from build123d import *

# Parameters (mm, degrees)
SALIENTE_EXTRUIR1_DEPTH      = 5
SALIENTE_EXTRUIR1_DEPTH_BACK = 5
SALIENTE_EXTRUIR2_START      = 14
CROQUIS2_R                   = 5
SALIENTE_EXTRUIR2_DEPTH      = 10
CROQUIS4_W                   = 10
CROQUIS4_H                   = 2.771281292
SALIENTE_EXTRUIR3_DEPTH      = 18.9
CHAFL_N1_SIZE                = 1.2
CROQUIS5_R                   = 1.7
CORTAR_EXTRUIR1_DEPTH        = 33.252493444
CROQUIS2_4_R                 = 5
SALIENTE_EXTRUIR8_DEPTH      = 14
CHAFL_N2_SIZE                = 10
CHAFL_N2_SIZE_2              = 1.3
CORTAR_EXTRUIR2_DEPTH        = 31.412223535
CORTAR_EXTRUIR2_DEPTH_BACK   = 31.412223535


# Some blends are built 0.0001 mm under size
with BuildPart() as part:
    # Croquis1 → Saliente-Extruir1 (new, two sides: drawn at the far end of the back side and taken through both)
    with BuildSketch(Plane(origin=(0, 0, 0), x_dir=(0, 0, -1), z_dir=(1, 0, 0)).offset(-SALIENTE_EXTRUIR1_DEPTH_BACK)):
        Polygon((2.829016319, 4.9), (-2.829016319, 4.9), (-5.658032638, 0), (-2.829016319, -4.9), (2.829016319, -4.9), (5.658032638, 0), align=None)
        Polygon((2.886751346, 0), (1.443375673, 2.5), (-1.443375673, 2.5), (-2.886751346, 0), (-1.443375673, -2.5), (1.443375673, -2.5), align=None, mode=Mode.SUBTRACT)
    extrude(amount=SALIENTE_EXTRUIR1_DEPTH + SALIENTE_EXTRUIR1_DEPTH_BACK)



with BuildPart() as body_2:
    # Croquis2 → Saliente-Extruir2 (new body)
    with BuildSketch(Plane(origin=(0, 4.9, 0), x_dir=(1, 0, 0), z_dir=(0, 1, 0)).offset(SALIENTE_EXTRUIR2_START)):
        Polygon((0, 7.159143338), (-6.2, 3.579571669), (-6.2, -3.579571669), (0, -7.159143338), (6.2, -3.579571669), (6.2, 3.579571669), align=None)
        with Locations(Location((0, 0, 0), (0, 0, 270))):
            Circle(CROQUIS2_R, mode=Mode.SUBTRACT)
    extrude(amount=SALIENTE_EXTRUIR2_DEPTH)


with BuildPart() as part_1:
    add(part.part)

    add(body_2.part)  # Saliente-Extruir3 merges body 2
    # Croquis4 → Saliente-Extruir3 (add)
    with BuildSketch(Plane(origin=(0, 0, 0), x_dir=(1, 0, 0), z_dir=(0, 1, 0))):
        with Locations((0, -4.272391992)):
            Rectangle(CROQUIS4_W, CROQUIS4_H)
        with Locations((0, 4.272391992)):
            Rectangle(CROQUIS4_W, CROQUIS4_H)
    extrude(amount=SALIENTE_EXTRUIR3_DEPTH)

    # Chaflán1
    chafl_n1_edges = [part_1.edges().sort_by_distance(p)[0] for p in [
        (3.8, 18.9, 4.965212315),
        (-3.8, 18.9, 4.965212315),
        (-3.8, 18.9, -4.965212315),
        (3.8, 18.9, -4.965212315),
    ]]
    chamfer(chafl_n1_edges, length=CHAFL_N1_SIZE - 0.0001)  # a hair under: the kernel refuses the full size

    # Croquis5 → Cortar-Extruir1 (cut, through all)
    with BuildSketch(Plane(origin=(6.2, 0, 0), x_dir=(0, 0, -1), z_dir=(1, 0, 0))):
        with Locations((0, 23.9)):
            Circle(CROQUIS5_R)
    extrude(amount=-CORTAR_EXTRUIR1_DEPTH, mode=Mode.SUBTRACT)

    # Croquis2<4> → Saliente-Extruir8 (add)
    # profile 1 of 2: a face of its own
    with BuildSketch(Plane(origin=(0, 4.9, 0), x_dir=(1, 0, 0), z_dir=(0, 1, 0))):
        Polygon((6.2, -3.579571669), (6.2, 3.579571669), (0, 7.159143338), (-6.2, 3.579571669), (-6.2, -3.579571669), (0, -7.159143338), align=None)
        with Locations(Location((0, 0, 0), (0, 0, 270))):
            Circle(CROQUIS2_4_R, mode=Mode.SUBTRACT)
    # profile 2 of 2: a face of its own
    with BuildSketch(Plane(origin=(0, 4.9, 0), x_dir=(1, 0, 0), z_dir=(0, 1, 0))):
        with Locations(Location((0, 0, 0), (0, 0, 270))):
            Circle(CROQUIS2_4_R)
    extrude(amount=SALIENTE_EXTRUIR8_DEPTH)

    # Chaflán2
    # the kernel refuses this chamfer: 10, 1.3 mm, written as the material it takes off along each edge
    with BuildSketch(Plane(origin=(-25.109710919, 4.9, -7.33795502), x_dir=(-0.00247990444519022, 0.9999877000722412, 0.004295320496985479), z_dir=(0.8660254037844387, 0, 0.5000000000000001))) as chafl_n2_piece_1_section:
        Polygon((CHAFL_N2_SIZE * 0.999987700072, -CHAFL_N2_SIZE * 0.00495980889038), (-CHAFL_N2_SIZE_2 * 0.00495980889038, -CHAFL_N2_SIZE_2 * 0.999987700072), (0, 0), align=None)
    chafl_n2_piece_1 = extrude(amount=54.986172033, mode=Mode.PRIVATE)
    chafl_n2_piece_1 = split(chafl_n2_piece_1, bisect_by=Plane(origin=(-0.715, 8.4, 5.658032638), z_dir=(0, 0, 1)), keep=Keep.TOP, mode=Mode.PRIVATE)
    add(chafl_n2_piece_1, mode=Mode.SUBTRACT)
    with BuildSketch(Plane(origin=(-22.509710919, 4.9, 20.155130996), x_dir=(-0.47976503705991164, -0.28160617333362153, -0.8309774198829328), z_dir=(0.8660254037844388, 0, -0.49999999999999967))) as chafl_n2_piece_2_section:
        Polygon((CHAFL_N2_SIZE_2 * 0.95953007412, CHAFL_N2_SIZE_2 * 0.281606173334), (-CHAFL_N2_SIZE * 0.281606173334, CHAFL_N2_SIZE * 0.95953007412), (0, 0), align=None)
    chafl_n2_piece_2 = extrude(amount=54.986172033, mode=Mode.PRIVATE)
    chafl_n2_piece_2 = split(chafl_n2_piece_2, bisect_by=Plane(origin=(0.715, 8.4, 5.658032638), z_dir=(0, 0, 1)), keep=Keep.TOP, mode=Mode.PRIVATE)
    add(chafl_n2_piece_2, mode=Mode.SUBTRACT)
    with BuildSketch(Plane(origin=(22.509710919, 4.9, -20.155130996), x_dir=(-0.002479904445190118, 0.9999877000722412, -0.004295320496985084), z_dir=(-0.8660254037844387, 0, 0.49999999999999994))) as chafl_n2_piece_3_section:
        Polygon((CHAFL_N2_SIZE * 0.999987700072, -CHAFL_N2_SIZE * 0.00495980889038), (-CHAFL_N2_SIZE_2 * 0.00495980889038, -CHAFL_N2_SIZE_2 * 0.999987700072), (0, 0), align=None)
    chafl_n2_piece_3 = extrude(amount=54.986172033, mode=Mode.PRIVATE)
    chafl_n2_piece_3 = split(chafl_n2_piece_3, bisect_by=Plane(origin=(-0.715, 8.4, -5.658032638), z_dir=(0, 0, -1)), keep=Keep.TOP, mode=Mode.PRIVATE)
    add(chafl_n2_piece_3, mode=Mode.SUBTRACT)
    with BuildSketch(Plane(origin=(25.109710919, 4.9, 7.33795502), x_dir=(-0.4797650370599119, -0.28160617333362137, 0.8309774198829327), z_dir=(-0.8660254037844387, 0, -0.5000000000000001))) as chafl_n2_piece_4_section:
        Polygon((CHAFL_N2_SIZE_2 * 0.95953007412, CHAFL_N2_SIZE_2 * 0.281606173334), (-CHAFL_N2_SIZE * 0.281606173334, CHAFL_N2_SIZE * 0.95953007412), (0, 0), align=None)
    chafl_n2_piece_4 = extrude(amount=54.986172033, mode=Mode.PRIVATE)
    chafl_n2_piece_4 = split(chafl_n2_piece_4, bisect_by=Plane(origin=(0.715, 8.4, -5.658032638), z_dir=(0, 0, -1)), keep=Keep.TOP, mode=Mode.PRIVATE)
    add(chafl_n2_piece_4, mode=Mode.SUBTRACT)

    # Croquis6 → Cortar-Extruir2 (cut, two sides: drawn at the far end of the back side and taken through both)
    with BuildSketch(Plane.XY.offset(-CORTAR_EXTRUIR2_DEPTH_BACK)):
        Polygon((5, 14.9), (6.2, 16.9), (6.2, 4.9), (5, 4.9), align=None)
        Polygon((-6.2, 4.9), (-5, 4.9), (-5, 14.9), (-6.2, 16.9), align=None)
    extrude(amount=CORTAR_EXTRUIR2_DEPTH + CORTAR_EXTRUIR2_DEPTH_BACK, mode=Mode.SUBTRACT)


solid = part_1.part
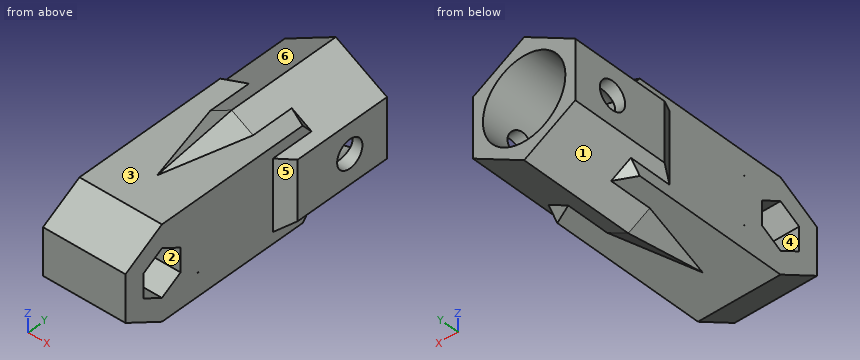
Read the model definition and answer for the solid it produces. Units are mm, in the model's axes. Face numbers are marked on the shaded views. A direction names the side the tool comes from. Round coordinates to 2 decimals unless told otherwise and drop trailing zeros. Write each loop counter-clockwise with the first axis right and the second up, starting at its lowest first coordinate (ties: lowest second). Pieces come first, ordered by that corner, then holes. Notation, with made-up numbers: M -9.75,23.25 L 40.25,23.25 A28 ccw 40.25,56.25 Z; hole C 3.25,81.25 d10. An arc over 180 degrees is marked long. Use a Markdown table: item, result.
1) For a pull along Z with two mould halves and no side action, classify the marked faces 4, 5 and 6 as pulls with the +Z half, pulls with the -Z half, needs draft (parallel to the pull), parting line crosses it, or undercut.
Answers follow:
| item | result |
|---|---|
| face 4 | undercut |
| face 5 | needs draft |
| face 6 | pulls with the +Z half |
2) The part is cut by section A-A (z = 0). Write down the section's boundary in (x, y).
Answers follow:
| item | result |
|---|---|
| outline | M -6.2,16.9 L -5,14.9 L -5,2.5 L 5,2.5 L 5,14.9 L 6.2,16.9 L 6.2,22.2 L 5,22.2 L 5,18.9 L -5,18.9 L -5,22.2 L -6.2,22.2 Z; M -6.2,25.6 L -5,25.6 L -5,28.9 L -6.2,28.9 Z; M -5,-4.9 L 5,-4.9 L 5,-2.5 L -5,-2.5 Z; M 5,25.6 L 6.2,25.6 L 6.2,28.9 L 5,28.9 Z |
3) The part is cut by section D-D (y = 10). Write down the section's boundary in (x, z), plus the area to 3 significant figures.
Answers follow:
| item | result |
|---|---|
| outline | M -5,-5.66 L -1.33,-5.66 L 0,-6.42 L 1.33,-5.66 L 5,-5.66 L 5,5.66 L 1.33,5.66 L 0,6.42 L -1.33,5.66 L -5,5.66 Z |
| area | 115 mm2 |
4) A tool of negligible diameter and unlimited length cuts with its end or side. For the marked faces 1, 2 and 3, from which of +Z, -Z, +X, -X, +Y, -Y can it reach the whole face along a straight path? Write none if from no direction.
Answers follow:
| item | result |
|---|---|
| face 1 | -Z, -X, +Y |
| face 2 | +X, -X |
| face 3 | +Z, -Y |
5) The part is cut by section C-C (x = -3.75). Write down the section's boundary in (y, z).
Answers follow:
| item | result |
|---|---|
| outline | M -4.9,-2.83 L 0,-5.66 L 19.52,-5.66 L 20.1,-4.99 L 28.9,-4.99 L 28.9,-3.31 L 18.9,-3.31 L 18.9,3.31 L 28.9,3.31 L 28.9,4.99 L 20.1,4.99 L 19.52,5.66 L 0,5.66 L -4.9,2.83 Z; hole M -2.5,-1.44 L 0,-2.89 L 2.5,-1.44 L 2.5,1.44 L 0,2.89 L -2.5,1.44 Z; hole M 4.8,-2.89 L 4.9,-2.89 L 4.9,-2.83 Z; hole M 4.8,2.89 L 4.9,2.83 L 4.9,2.89 Z |
6) Flat-ended cylindrical pins translate along their axes: pin 1 (5 mm diameter, centred on x = 3, y = 15.5, fed in from +Z); pin 2 (2 mm diameter, centred on x = 2.5, y = 11.5, fed in from +Z); pin 3 (2.5 mm diameter, centred on x = -1, z = -0.5, fed in from +Y); pin 4 (2.5 mm diameter, centred on y = 23.9, z = 0, fed in from -X). Find the tip coordinate at first contact, or state that the pin passes through.
Answers follow:
| item | result |
|---|---|
| pin 1 | stops at z = 6.87 |
| pin 2 | stops at z = 5.8 |
| pin 3 | stops at y = 18.9 |
| pin 4 | passes through |
7) Straight lines are drawn through the part: line 1 along Y through (x, z) = (-2.25, -0.25); line 2 along X through (y, z) = (18, -4.5); line 3 along X through (y, z) = (22, 0). For each, find the intervals that lie inside material, in ascending order. Write a range as [from, to].
Answers follow:
| item | result |
|---|---|
| line 1 | y = [-4.9, -2.5], [2.5, 18.9] |
| line 2 | x = [-5, 5] |
| line 3 | x = [-6.2, -5], [5, 6.2] |
8) The part is cut by section B-B (y = 26.5). Write down the section's boundary in (x, z).
Answers follow:
| item | result |
|---|---|
| outline | M -6.2,-3.58 L 0,-7.16 L 6.2,-3.58 L 6.2,3.58 L 0,7.16 L -6.2,3.58 Z; hole C 0,0 d10 |
